from build123d import *

# Parameters (mm, degrees)
SKETCH_1_W           = 70
SKETCH_1_H           = 45.4
EXTRUDE_1_DEPTH      = 2.2
SKETCH_2_R           = 1.62
CUT_EXTRUDE_1_DEPTH  = 12.2
SKETCH_3_W           = 29
SKETCH_3_H           = 17.6
CUT_EXTRUDE_2_DEPTH  = 12.2
SKETCH_5_R           = 1.07
SKETCH_5_R_2         = 3
CUT_EXTRUDE_4_DEPTH  = 12.2
SKETCH_6_W           = 53
SKETCH_6_H           = 6.3
CUT_EXTRUDE_5_DEPTH  = 12.2
SKETCH_7_W           = 75.7
SKETCH_7_H           = 2
EXTRUDE_3_DEPTH      = 22
SKETCH_8_W           = 2
SKETCH_8_H           = 49.4
EXTRUDE_4_DEPTH      = 22
SKETCH_9_W           = 75.7
SKETCH_9_H           = 2
EXTRUDE_5_DEPTH      = 22
SKETCH_10_W          = 5.7
SKETCH_10_H          = 45.4
EXTRUDE_6_DEPTH      = 2.2
SKETCH_11_W          = 2
SKETCH_11_H          = 49.4
EXTRUDE_7_DEPTH      = 22
SKETCH_12_W          = 20
SKETCH_12_H          = 10
CUT_EXTRUDE_6_DEPTH  = 22
SKETCH_13_W          = 32
SKETCH_13_H          = 6
CUT_EXTRUDE_7_DEPTH  = 22
SKETCH_14_W          = 30
SKETCH_14_H          = 10
CUT_EXTRUDE_8_DEPTH  = 22
SKETCH_16_W          = 70
SKETCH_16_H          = 10
CUT_EXTRUDE_9_DEPTH  = 22
SKETCH_17_W          = 48.7
SKETCH_17_H          = 4
EXTRUDE_8_DEPTH      = 1.2
SKETCH_18_W          = 7
SKETCH_18_H          = 4
EXTRUDE_9_DEPTH      = 1.2
CUT_EXTRUDE_10_DEPTH = 11.2


with BuildPart() as part:
    # 草图1 → 凸台-拉伸1 (new body)
    with BuildSketch(Plane(origin=(0, 0, 0), x_dir=(1, 0, 0), z_dir=(0, 1, 0))):
        Rectangle(SKETCH_1_W, SKETCH_1_H)
    extrude(amount=EXTRUDE_1_DEPTH)

    # 草图2 → 切除-拉伸1 (cut)
    with BuildSketch(Plane(origin=(0, 2.2, 0), x_dir=(1, 0, 0), z_dir=(0, 1, 0))):
        with Locations(Location((-30.4, 18.05, 0), (0, 0, 270))):
            Circle(SKETCH_2_R)
        with Locations(Location((-30.4, -17.85, 0), (0, 0, 270))):
            Circle(SKETCH_2_R)
        with Locations(Location((30.4, -17.85, 0), (0, 0, 270))):
            Circle(SKETCH_2_R)
        with Locations(Location((30.4, 18.05, 0), (0, 0, 270))):
            Circle(SKETCH_2_R)
    extrude(amount=-CUT_EXTRUDE_1_DEPTH, mode=Mode.SUBTRACT)

    # 草图3 → 切除-拉伸2 (cut)
    with BuildSketch(Plane(origin=(0, 2.2, 0), x_dir=(1, 0, 0), z_dir=(0, 1, 0))):
        with Locations((-1.5, -2.1)):
            Rectangle(SKETCH_3_W, SKETCH_3_H)
    extrude(amount=-CUT_EXTRUDE_2_DEPTH, mode=Mode.SUBTRACT)

    # 草图5 → 切除-拉伸4 (cut)
    with BuildSketch(Plane(origin=(0, 2.2, 0), x_dir=(1, 0, 0), z_dir=(0, 1, 0))):
        with Locations(Location((9, 15.2, 0), (0, 0, 270))):
            Circle(SKETCH_5_R)
        with Locations(Location((-9, 15.2, 0), (0, 0, 270))):
            Circle(SKETCH_5_R)
        with Locations(Location((0, 15.2, 0), (0, 0, 270))):
            Circle(SKETCH_5_R_2)
    extrude(amount=-CUT_EXTRUDE_4_DEPTH, mode=Mode.SUBTRACT)

    # 草图6 → 切除-拉伸5 (cut)
    with BuildSketch(Plane(origin=(0, 2.2, 0), x_dir=(1, 0, 0), z_dir=(0, 1, 0))):
        with Locations((0, -17.45)):
            Rectangle(SKETCH_6_W, SKETCH_6_H)
    extrude(amount=-CUT_EXTRUDE_5_DEPTH, mode=Mode.SUBTRACT)

    # 草图7 → 凸台-拉伸3 (add)
    with BuildSketch(Plane(origin=(0, 2.2, 0), x_dir=(1, 0, 0), z_dir=(0, 1, 0))):
        with Locations((-2.85, 23.7)):
            Rectangle(SKETCH_7_W, SKETCH_7_H)
    extrude(amount=-EXTRUDE_3_DEPTH)

    # 草图8 → 凸台-拉伸4 (add)
    with BuildSketch(Plane(origin=(0, 2.2, 0), x_dir=(1, 0, 0), z_dir=(0, 1, 0))):
        with Locations((36, 0)):
            Rectangle(SKETCH_8_W, SKETCH_8_H)
    extrude(amount=-EXTRUDE_4_DEPTH)

    # 草图9 → 凸台-拉伸5 (add)
    with BuildSketch(Plane(origin=(0, 2.2, 0), x_dir=(1, 0, 0), z_dir=(0, 1, 0))):
        with Locations((-2.85, -23.7)):
            Rectangle(SKETCH_9_W, SKETCH_9_H)
    extrude(amount=-EXTRUDE_5_DEPTH)

    # 草图10 → 凸台-拉伸6 (add)
    with BuildSketch(Plane(origin=(0, 2.2, 0), x_dir=(1, 0, 0), z_dir=(0, 1, 0))):
        with Locations((-37.85, 0)):
            Rectangle(SKETCH_10_W, SKETCH_10_H)
    extrude(amount=-EXTRUDE_6_DEPTH)

    # 草图11 → 凸台-拉伸7 (add)
    with BuildSketch(Plane(origin=(0, 2.2, 0), x_dir=(1, 0, 0), z_dir=(0, 1, 0))):
        with Locations((-41.7, 0)):
            Rectangle(SKETCH_11_W, SKETCH_11_H)
    extrude(amount=-EXTRUDE_7_DEPTH)

    # 草图12 → 切除-拉伸6 (cut)
    with BuildSketch(Plane.XY.offset(24.7)):
        with Locations((18, -14.8)):
            Rectangle(SKETCH_12_W, SKETCH_12_H)
    extrude(amount=-CUT_EXTRUDE_6_DEPTH, mode=Mode.SUBTRACT)

    # 草图13 → 切除-拉伸7 (cut)
    with BuildSketch(Plane.ZY.offset(42.7)):
        with Locations((0, -16.8)):
            Rectangle(SKETCH_13_W, SKETCH_13_H)
    extrude(amount=-CUT_EXTRUDE_7_DEPTH, mode=Mode.SUBTRACT)

    # 草图14 → 切除-拉伸8 (cut)
    with BuildSketch(Plane(origin=(37, 0, 0), x_dir=(0, 0, -1), z_dir=(1, 0, 0))):
        with Locations((0, -8.8)):
            Rectangle(SKETCH_14_W, SKETCH_14_H)
    extrude(amount=-CUT_EXTRUDE_8_DEPTH, mode=Mode.SUBTRACT)

    # 草图16 → 切除-拉伸9 (cut)
    with BuildSketch(Plane(origin=(0, 0, -24.7), x_dir=(-1, 0, 0), z_dir=(0, 0, -1))):
        with Locations((2.85, -5.8)):
            Rectangle(SKETCH_16_W, SKETCH_16_H)
    extrude(amount=-CUT_EXTRUDE_9_DEPTH, mode=Mode.SUBTRACT)

    # 草图17 → 凸台-拉伸8 (add)
    with BuildSketch(Plane(origin=(0, 0, 22.7), x_dir=(-1, 0, 0), z_dir=(0, 0, -1))):
        with Locations((16.35, -17.8)):
            Rectangle(SKETCH_17_W, SKETCH_17_H)
    extrude(amount=EXTRUDE_8_DEPTH)

    # 草图18 → 凸台-拉伸9 (add)
    with BuildSketch(Plane(origin=(0, 0, 22.7), x_dir=(-1, 0, 0), z_dir=(0, 0, -1))):
        with Locations((-31.5, -17.8)):
            Rectangle(SKETCH_18_W, SKETCH_18_H)
    extrude(amount=EXTRUDE_9_DEPTH)

    # 草图19 → 切除-拉伸10 (cut)
    with BuildSketch(Plane(origin=(0, 2.2, 0), x_dir=(1, 0, 0), z_dir=(0, 1, 0))):
        Polygon((22.919485098, -4.254171533), (19.344175277, -6.13844673), (15.924690179, -3.984275197), (16.080514902, 0.054171533), (19.655824723, 1.93844673), (23.075309821, -0.215724803), align=None)
        Polygon((-19.080514902, 0.054171533), (-22.655824723, 1.93844673), (-26.075309821, -0.215724803), (-25.919485098, -4.254171533), (-22.344175277, -6.13844673), (-18.924690179, -3.984275197), align=None)
    extrude(amount=-CUT_EXTRUDE_10_DEPTH, mode=Mode.SUBTRACT)


solid = part.part
For this review, take the finished solid that the model builds, in its own axes (mm). A direction names the side the tool comes from. Round coordinates to 2 decimals unless told otherwise and drop trailing zeros. Loops run counter-clockwise (first coordinate to the right, second up) from the corner with the lowest first, then second, coordinate; pieces in that order, holes last. Notation, with made-up numbers: (49.25, -36.5) - (108.25, -36.5) arc R12 cw to (108.25, -16.5) - close; hole circle Ø11 at (88, 44). An arc over 180 degrees is marked (long way). Answer as CSV lines item,"result".
(1) Consider section A-A on y = -8.5. Give the boundary of the cut face in (x, z), then the cut area to 3 significant figures.
Checked values:
outline,"(-42.7, -24.7) - (-37.85, -24.7) - (-37.85, -22.7) - (-40.7, -22.7) - (-40.7, 22.7) - (35, 22.7) - (35, 15) - (37, 15) - (37, 24.7) - (-42.7, 24.7) - close; (32.15, -24.7) - (37, -24.7) - (37, -15) - (35, -15) - (35, -22.7) - (32.15, -22.7) - close"
area,"300 mm2"
(2) Tool access review of faces 4 (the face through (-42, -17, -16)), 5 (the face through (-3, -16, -22.7)), 6 (the face through (-19, -19.8, 23)), 7 (the face through (16, 1, 2)), 8 (the face through (36, -9, 15)): name each direction out of +Z, -Z, +X, -X, +Y, -Y from which nothing blocks a thin tool from reaching the whole face with its end or side.
Checked values:
face 4,"-X, -Y"
face 5,"-Y"
face 6,"+Z, -Z, +X, -X, -Y"
face 7,"+Y, -Y"
face 8,"+X"
(3) Mouldability with a two-part tool opening along Z and no side actions: class faces 1 (the face through (28.963, 1.115, 18.598)), 2 (the face through (-24.16, 1.12, 5.18)), 3 (the face through (37, -1, 0)) as +Z half, -Z half, draft (parallel to the pull), parting line (faces both ways), or undercut.
Checked values:
face 1,"undercut"
face 2,"undercut"
face 3,"draft"
(4) Consider section C-C on x = 5. Give the boundary of the cut face in (y, z).
Checked values:
outline,"(-19.8, -24.7) - (-10.8, -24.7) - (-10.8, -22.7) - (-19.8, -22.7) - close; (-19.8, 21.5) - (-15.8, 21.5) - (-15.8, 22.7) - (0, 22.7) - (0, 20.6) - (2.2, 20.6) - (2.2, 24.7) - (-19.8, 24.7) - close; (-0.8, -24.7) - (2.2, -24.7) - (2.2, -6.7) - (0, -6.7) - (0, -22.7) - (-0.8, -22.7) - close; (0, 10.9) - (2.2, 10.9) - (2.2, 14.3) - (0, 14.3) - close"
(5) Consider section B-B on z = 17.85. Give the boundary of the cut face in (x, y).
Checked values:
outline,"(-42.7, -19.8) - (-40.7, -19.8) - (-40.7, 0) - (-32.02, 0) - (-32.02, 2.2) - (-42.7, 2.2) - close; (-28.78, 0) - (-26.5, 0) - (-26.5, 2.2) - (-28.78, 2.2) - close; (26.5, 0) - (28.78, 0) - (28.78, 2.2) - (26.5, 2.2) - close; (32.02, 0) - (35, 0) - (35, -19.8) - (37, -19.8) - (37, 2.2) - (32.02, 2.2) - close"
(6) Consider section D-D on x = -9. Give the boundary of the cut face in (y, z).
Checked values:
outline,"(-19.8, -24.7) - (-10.8, -24.7) - (-10.8, -22.7) - (-19.8, -22.7) - close; (-19.8, 21.5) - (-15.8, 21.5) - (-15.8, 22.7) - (0, 22.7) - (0, 20.6) - (2.2, 20.6) - (2.2, 24.7) - (-19.8, 24.7) - close; (-0.8, -24.7) - (2.2, -24.7) - (2.2, -16.27) - (0, -16.27) - (0, -22.7) - (-0.8, -22.7) - close; (0, -14.13) - (2.2, -14.13) - (2.2, -6.7) - (0, -6.7) - close; (0, 10.9) - (2.2, 10.9) - (2.2, 14.3) - (0, 14.3) - close"
(7) Wall thickness on line 1 (X direction, y = 0.5, z = 17.85); line 2 (Z direction, x = 31, y = -18.75); line 3 (X direction, y = -2, z = 4.5): over which ranges is each line inside the solid? List them lowest first.
Checked values:
line 1,"x = -42.7 to -32.02, -28.78 to -26.5, 26.5 to 28.78, 32.02 to 37"
line 2,"z = -24.7 to -22.7, 21.5 to 24.7"
line 3,"x = -42.7 to -40.7, 35 to 37"
(8) Insertion check: P1, Ø1.5, axis at x = -14, z = 19.5, coming from the -Y side; P2, Ø3, axis at x = 7, z = 19.5, coming from the -Y side; P3, Ø0.6, axis at x = 13.5, z = 23.5, coming from the -Y side. Each pin has a flat end and moves straight along its axis. Give the tip position at first contact, or say it passes through.
Checked values:
P1,"passes through"
P2,"stops at y = 0"
P3,"stops at y = -9.8"
